Autodesk Inventor part; units mm, degrees
ref_plane "YZ Plane" through (0, 0, 0) normal (1, 0, 0) x (0, 1, 0)
ref_plane "XZ Plane" through (0, 0, 0) normal (0, 1, 0) x (-1, 0, 0)
ref_plane "XY Plane" through (0, 0, 0) normal (0, 0, 1) x (1, 0, 0)
sketch "Эскиз1" plane through (0, 0, 0) normal (0, 0, 1) x (1, 0, 0)
  line L0 (0, 3.25) -> (0, -3.25)
  line L1 (0, -2.25) -> (33.5687, -2.25)
  line L2 (35.2894, -1.7075) -> (41.8528, 2.8883)
  line L3 (45, 1.25) -> (45, -3.25)
  arc A0 (33.5687, -2.25) -> (35.2894, -1.7075) centre (33.5687, 0.75) ccw
  arc A1 (45, 1.25) -> (41.8528, 2.8883) centre (43, 1.25) ccw
  line L4 (0, 3.25) -> (45, 3.25) construction
  line L5 (0, -3.25) -> (33.2828, -3.25)
  line L6 (35.0035, -2.7075) -> (40.8528, 1.3883)
  line L7 (44, -0.25) -> (44, -3.25)
  arc A2 (33.2828, -3.25) -> (35.0035, -2.7075) centre (33.2828, -0.25) ccw
  arc A3 (44, -0.25) -> (40.8528, 1.3883) centre (42, -0.25) ccw
  line L8 (44, -3.25) -> (45, -3.25)
  point P0 (0, 0)
  point P1 (0, 0)
  dimension "d0" = 6.5
  dimension "d1" = 1
  dimension "d2" = 3
  dimension "d3" = 55
  dimension "d4" = 90
  dimension "d5" = 2
  dimension "d6" = 55
  dimension "d7" = 3
  dimension "d8" = 2
  dimension "d9" = 1
revolve "Вращение1" add sketch "Эскиз1" angle 360 about axis through (0, 3.25, 0) along (0, -1, 0)
properties part number "77. Заглушка"
Check sheet for the modelled part. Datum: model origin and axes. Units: mm. A direction names the side the tool comes from. Give positions to 0.01 mm unless a question says otherwise; leave off trailing zeros. Order: outer loops, then holes, each group sorted by start corner. A loop starts at its lowest first (then second) coordinate and runs counter-clockwise, first axis right, second up. Notation, with made-up numbers: M 72,63.25 L 109,63.25 A22 cw 109,93.25 Z; hole C 32.5,87.25 d4. An arc over 180 degrees is marked long. Answer in a Markdown table with one row per item. Add a question column.
Q1. Gauge pin test, flat ends, axial feed: pin 1 Ø1 at (x, z) = (-22.5, 8) entering from +Y; pin 2 Ø3 at (x, z) = (-34, -14) entering from +Y; pin 3 Ø1.5 at (x, z) = (32.5, 11) entering from -Y. Record the tip position at first contact, or that the pin passes through.
Q2. Sectioned sample at A-A, the plane z = 0. Record the boundary of the cut face in (x, y).
Q3. Access from +Z, -Z, +X, -X, +Y, -Y to the whole of each face (thin tool, end or side, straight path). Record for faces 1 (the conical face through (16.32, -2.45, 31.38)), 2 (the flat face through (0, -2.25, 0)).
Q4. Release check for a two-part mould opening along Z. For faces 3 (the cylindrical face through (-9.538, -1.771, -42.954)), 4 (the flat face through (0, -3.25, 0)), 5 (the cylindrical face through (20.765, -1.031, -39.923)) record: released by +Z, released by -Z, zero draft, split by the parting line, or undercut.
Q5. Sectioned sample at B-B, the plane x = 0. Record the boundary of the cut face in (y, z).
Q6. Thickness scan on L1, parallel to X at y = -1.5, z = 6; L2, parallel to Z at x = 0, y = -1.45; L3, parallel to Z at x = 0, y = -1.85. Record the ranges inside material, lowest first.
Verdict:
| question | item | result |
|---|---|---|
| 1 | pin 1 | y = -2.25 |
| 1 | pin 2 | y = 0.38 |
| 1 | pin 3 | y = -3.24 |
| 2 | outline | M -45,-3.25 L -44,-3.25 L -44,-0.25 A2 cw -40.85,1.39 L -35,-2.71 A3 ccw -33.28,-3.25 L 33.28,-3.25 A3 ccw 35,-2.71 L 40.85,1.39 A2 cw 44,-0.25 L 44,-3.25 L 45,-3.25 L 45,1.25 A2 ccw 41.85,2.89 L 35.29,-1.71 A3 cw 33.57,-2.25 L -33.57,-2.25 A3 cw -35.29,-1.71 L -41.85,2.89 A2 ccw -45,1.25 Z |
| 3 | face 1 | -Y |
| 3 | face 2 | +Y |
| 4 | face 3 | undercut |
| 4 | face 4 | zero draft |
| 4 | face 5 | split by the parting line |
| 5 | outline | M -3.25,-45 L 1.25,-45 A2 ccw 2.89,-41.85 L -1.71,-35.29 A3 cw -2.25,-33.57 L -2.25,33.57 A3 cw -1.71,35.29 L 2.89,41.85 A2 ccw 1.25,45 L -3.25,45 L -3.25,44 L -0.25,44 A2 cw 1.39,40.85 L -2.71,35 A3 ccw -3.25,33.28 L -3.25,-33.28 A3 ccw -2.71,-35 L 1.39,-40.85 A2 cw -0.25,-44 L -3.25,-44 Z |
| 6 | L1 | -44.6 to -43.59, -36.23 to -35.08, 35.08 to 36.23, 43.59 to 44.6 |
| 6 | L2 | -45 to -44, -36.8 to -35.66, 35.66 to 36.8, 44 to 45 |
| 6 | L3 | -45 to -44, -36.23 to -35.07, 35.07 to 36.23, 44 to 45 |
